Input: part model. Units: mm. Frame: model coordinates. Give positions to 0.01 mm unless a question says otherwise; leave off trailing zeros. Order: outer loops, then holes, each group sorted by start corner. A loop starts at its lowest first (then second) coordinate and runs counter-clockwise, first axis right, second up. Notation, with made-up numbers: (62.25, -40) - (88.25, -40) arc R9 cw to (88.25, -23) - close; hole circle Ø5 at (63, 56). An arc over 180 degrees is marked (long way). Answer in a Markdown table with one row per item. Add a question column.
from build123d import *

# Parameters (mm, degrees)
F0_R     = 6
F1_DEPTH = 6
F3_DEPTH = 2714.7
F5_DEPTH = 120.001


with BuildPart() as f1:
    # F0 (on Top) → F1 (new body)
    with BuildSketch(Plane.XY):
        with BuildLine():
            ThreePointArc((90, 80), (87.071068, 87.071068), (80, 90))
            Line((80, 90), (-80, 90))
            ThreePointArc((-80, 90), (-87.071068, 87.071068), (-90, 80))
            Line((-90, 80), (-90, -80))
            ThreePointArc((-90, -80), (-87.071068, -87.071068), (-80, -90))
            Line((-80, -90), (80, -90))
            ThreePointArc((80, -90), (87.071068, -87.071068), (90, -80))
            Line((90, -80), (90, 80))
        make_face()
        with Locations((-65, -65)):
            Circle(F0_R, mode=Mode.SUBTRACT)
        with Locations((65, -65)):
            Circle(F0_R, mode=Mode.SUBTRACT)
        with Locations((-65, 65)):
            Circle(F0_R, mode=Mode.SUBTRACT)
        with Locations((65, 65)):
            Circle(F0_R, mode=Mode.SUBTRACT)
    extrude(amount=F1_DEPTH)

    # F2 (on face) → F3 (join)
    with BuildSketch(Plane.XY.offset(6)):
        with BuildLine():
            Line((-25, -30), (25, -30))
            ThreePointArc((25, -30), (28.535534, -28.535534), (30, -25))
            Line((30, -25), (30, 25))
            ThreePointArc((30, 25), (28.535534, 28.535534), (25, 30))
            Line((25, 30), (-25, 30))
            ThreePointArc((-25, 30), (-28.535534, 28.535534), (-30, 25))
            Line((-30, 25), (-30, -25))
            ThreePointArc((-30, -25), (-28.535534, -28.535534), (-25, -30))
        make_face()
        with BuildLine():
            ThreePointArc((25, 27), (26.414214, 26.414214), (27, 25))
            Line((27, 25), (27, -25))
            ThreePointArc((27, -25), (26.414214, -26.414214), (25, -27))
            Line((25, -27), (-25, -27))
            ThreePointArc((-25, -27), (-26.414214, -26.414214), (-27, -25))
            Line((-27, -25), (-27, 25))
            ThreePointArc((-27, 25), (-26.414214, 26.414214), (-25, 27))
            Line((-25, 27), (25, 27))
        make_face(mode=Mode.SUBTRACT)
    extrude(amount=F3_DEPTH)

    # F4 (on face) → F5 (cut, through all)
    with BuildSketch(Plane.XZ.offset(30)):
        Polygon((31.369732, 2720.7), (-30.02377, 2720.7), (31.369732, 2709.874669), align=None)
    extrude(amount=-F5_DEPTH, mode=Mode.SUBTRACT)


solid = f1.part
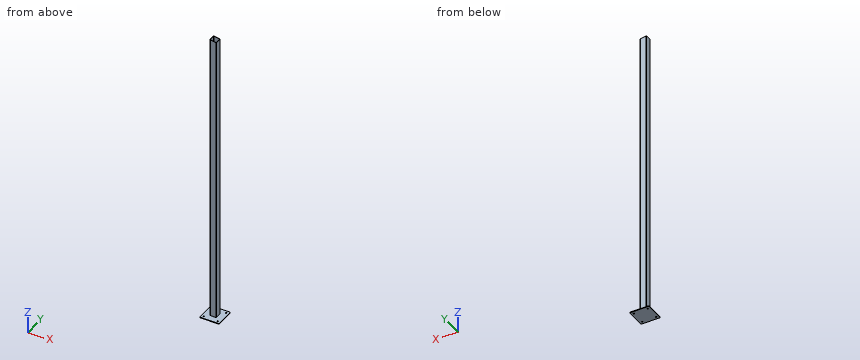
Q1. Section B-B, the plane y = -1.5. Return loops of the section in (x, z).
Q2. Section C-C, the plane x = 0.5. Return loops of the section in (y, z), then the cut area to 3 significant figures.
Q3. Contact query for flat-ended pins moving along their axis: P1, Ø15, axis at y = -11.5, z = 1543.5, coming from the +X side; P2, Ø25, axis at y = -8.5, z = 1353.5, coming from the -X side; P3, Ø6, axis at x = -23, z = 1431, coming from the +Y side; P4, Ø14, axis at x = 65, y = -65, coming from the -Z side. Output: stop coordinate, or through.
Q4. Section A-A, the plane z = 532. Return loops of the section in (x, y).
Q5. Line query: probe 1 along Y at (x, z) = (65, 2.2); probe 2 along Y at (x, z) = (-18.5, 1199.5). Output: solid intervals per line, ascending.
Computed:
| question | item | result |
|---|---|---|
| 1 | outline | (-90, 0) - (90, 0) - (90, 6) - (30, 6) - (30, 2710.12) - (27, 2710.65) - (27, 6) - (-27, 6) - (-27, 2720.17) - (-30, 2720.7) - (-30, 6) - (-90, 6) - close |
| 2 | outline | (-90, 0) - (90, 0) - (90, 6) - (30, 6) - (30, 2715.32) - (27, 2715.32) - (27, 6) - (-27, 6) - (-27, 2715.32) - (-30, 2715.32) - (-30, 6) - (-90, 6) - close |
| 2 | area | 17,300 mm^2 |
| 3 | P1 | stops at x = 30 |
| 3 | P2 | stops at x = -30 |
| 3 | P3 | stops at y = 30 |
| 3 | P4 | stops at z = 0 |
| 4 | outline | (-30, -25) arc R5 ccw to (-25, -30) - (25, -30) arc R5 ccw to (30, -25) - (30, 25) arc R5 ccw to (25, 30) - (-25, 30) arc R5 ccw to (-30, 25) - close; hole (-27, -25) arc R2 ccw to (-25, -27) - (25, -27) arc R2 ccw to (27, -25) - (27, 25) arc R2 ccw to (25, 27) - (-25, 27) arc R2 ccw to (-27, 25) - close |
| 5 | probe 1 | y = -90 to -71, -59 to 59, 71 to 90 |
| 5 | probe 2 | y = -30 to -27, 27 to 30 |
